from build123d import *

# Parameters (mm, degrees)
SKETCH_1_R          = 19
EXTRUDE_1_DEPTH     = 3
SKETCH_2_R          = 1.1
CUT_EXTRUDE_1_DEPTH = 37.891733491
CUT_EXTRUDE_2_DEPTH = 1.5
FILLET_1_R          = 1
FILLET_2_R          = 8


with BuildPart() as part:
    # Эскиз1 → Бобышка-Вытянуть1 (new body)
    with BuildSketch(Plane.XY):
        with BuildLine():
            Line((-26, 0), (-26, -26))
            Line((-26, -26), (26, -26))
            Line((26, -26), (26, 0))
            ThreePointArc((26, 0), (0, 26), (-26, 0))
        make_face()
        Circle(SKETCH_1_R, mode=Mode.SUBTRACT)
    extrude(amount=EXTRUDE_1_DEPTH)

    # Эскиз2 → Вырез-Вытянуть1 (cut, through all)
    with BuildSketch(Plane.XY.offset(3)):
        with Locations((0, 23.5)):
            Circle(SKETCH_2_R)
        with Locations((23.5, 0)):
            Circle(SKETCH_2_R)
        with Locations((0, -23.5)):
            Circle(SKETCH_2_R)
        with Locations((-23.5, 0)):
            Circle(SKETCH_2_R)
    extrude(amount=-CUT_EXTRUDE_1_DEPTH, mode=Mode.SUBTRACT)

    # Эскиз3 → Вырез-Вытянуть2 (cut)
    with BuildSketch(Plane.XY.offset(3)):
        with BuildLine():
            Line((-2, 23.5), (-2, 26))
            Line((-2, 26), (2, 26))
            Line((2, 26), (2, 23.5))
            ThreePointArc((2, 23.5), (0, 21.5), (-2, 23.5))
        make_face()
        with BuildLine():
            Line((26, -2), (23.5, -2))
            ThreePointArc((23.5, -2), (21.5, 0), (23.5, 2))
            Line((23.5, 2), (26, 2))
            Line((26, 2), (26, -2))
        make_face()
        with BuildLine():
            Line((-2, -26), (-2, -23.5))
            ThreePointArc((-2, -23.5), (0, -21.5), (2, -23.5))
            Line((2, -23.5), (2, -26))
            Line((2, -26), (-2, -26))
        make_face()
        with BuildLine():
            Line((-26, 2), (-23.5, 2))
            ThreePointArc((-23.5, 2), (-21.5, 0), (-23.5, -2))
            Line((-23.5, -2), (-26, -2))
            Line((-26, -2), (-26, 2))
        make_face()
    extrude(amount=-CUT_EXTRUDE_2_DEPTH, mode=Mode.SUBTRACT)

    # Скругление1
    fillet_1_edges = [part.edges().sort_by_distance(p)[0] for p in [
        (-25.922962794, 2, 2.25),
        (25.922962794, 2, 2.25),
        (2, 25.922962794, 2.25),
        (-2, 25.922962794, 2.25),
        (26, -2, 2.25),
        (2, -26, 2.25),
        (-2, -26, 2.25),
        (-26, -2, 2.25),
    ]]
    fillet(fillet_1_edges, radius=FILLET_1_R)

    # Скругление2
    fillet_2_edges = [part.edges().sort_by_distance(p)[0] for p in [
        (26, -26, 1.5),
        (-26, -26, 1.5),
    ]]
    fillet(fillet_2_edges, radius=FILLET_2_R)


solid = part.part
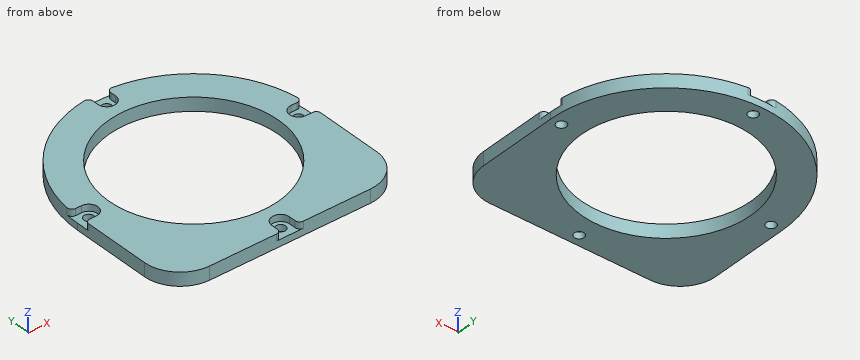
Can you work these out from the model? Positions are in its coordinate system, mm. Coordinates: 2 decimals unless noted, no trailing zeros. Write each loop counter-clockwise with the first axis right and the second up, starting at its lowest first coordinate (ties: lowest second). Pieces come first, ordered by that corner, then holes.
Q1. Imagine slicing it at A-A, the plane x = -14.5. List the corners of the cut face in (y, z) for me.
Results found:
outline: (-26, 0) - (-12.28, 0) - (-12.28, 3) - (-26, 3) - close; (12.28, 0) - (21.58, 0) - (21.58, 3) - (12.28, 3) - close
Q2. Imagine slicing it at C-C, the plane z = 0.75. List the corners of the cut face in (x, y) for me.
Results found:
outline: (-26, -18) arc R8 ccw to (-18, -26) - (18, -26) arc R8 ccw to (26, -18) - (26, 0) arc R26 ccw to (-26, 0) - close; hole circle Ø2.2 at (-23.5, 0); hole circle Ø38 at (0, 0); hole circle Ø2.2 at (0, -23.5); hole circle Ø2.2 at (0, 23.5); hole circle Ø2.2 at (23.5, 0)
Q3. For P1, Ø0.7, axis at x = -24.5, z = 2.5, coming from the -Y side; P2, Ø3, axis at x = 0, y = -23.5, coming from the +Z side; P3, Ø1, axis at y = 6.5, z = 2.5, coming from the +X side; P4, Ø3.5, axis at x = 23, y = 1.5, coming from the +Z side, each with a flat end and sliding along its axis, tell me the tip position at first contact or that it passes through.
Results found:
P1: stops at y = -23.12
P2: stops at z = 1.5
P3: stops at x = 25.3
P4: stops at z = 3
Q4. Imagine slicing it at B-B, the plane y = -7.5. List the corners of the cut face in (x, z) for me, plus the area to 3 significant figures.
Results found:
outline: (-26, 0) - (-17.46, 0) - (-17.46, 3) - (-26, 3) - close; (17.46, 0) - (26, 0) - (26, 3) - (17.46, 3) - close
area: 51.3 mm2
Q5. Please list where these lines run through material, in increasing order: L1, parallel to Y at x = 0, z = 0.7; L2, parallel to Y at x = -1, z = 1.15; L3, parallel to X at y = 12, z = 1.5.
Results found:
L1: y = -26 to -24.6, -22.4 to -19, 19 to 22.4, 24.6 to 26
L2: y = -26 to -23.96, -23.04 to -18.97, 18.97 to 23.04, 23.96 to 25.98
L3: x = -23.07 to -14.73, 14.73 to 23.07
